from build123d import *

# Parameters (mm, degrees)
F1_DEPTH = 508
F2_W     = 80.340108
F2_H     = 50.8
F2_W_2   = 82.870346
F3_DEPTH = 12.7
F4_W     = 83.715823
F4_H     = 50.8
F4_W_2   = 80.30174
F5_DEPTH = 12.7


with BuildPart() as f1:
    # F0 (on Front) → F1 (new body)
    with BuildSketch(Plane.XZ):
        with BuildLine():
            Line((3.550242, 42.501207), (-21.849758, 42.501207))
            ThreePointArc((-21.849758, 42.501207), (-32.272509, 23.451207), (-21.849758, 4.401207))
            Line((-21.849758, 4.401207), (3.550242, 4.401207))
            ThreePointArc((3.550242, 4.401207), (13.712078, 23.451207), (3.550242, 42.501207))
        make_face()
    extrude(amount=F1_DEPTH)

    # F2 (on face) → F3 (cut)
    with BuildSketch(Plane.XY.offset(42.501207)):
        with Locations((-9.149758, -406.4)):
            Rectangle(F2_W, F2_H)
        with Locations((-9.149758, -101.6)):
            Rectangle(F2_W_2, F2_H)
    extrude(amount=-F3_DEPTH, mode=Mode.SUBTRACT)

    # F4 (on face) → F5 (cut)
    with BuildSketch(Plane(origin=(0, 0, 4.401207), x_dir=(1, 0, 0), z_dir=(0, 0, -1))):
        with Locations((-9.149757, 101.6)):
            Rectangle(F4_W, F4_H)
        with Locations((-9.149758, 406.4)):
            Rectangle(F4_W_2, F4_H)
    extrude(amount=-F5_DEPTH, mode=Mode.SUBTRACT)


solid = f1.part
CAD build for the part. Positions are in the model's coordinates, mm. A direction names the side the tool comes from. Coordinates: 2 decimals unless noted, no trailing zeros. Loops run counter-clockwise (first coordinate to the right, second up) from the corner with the lowest first, then second, coordinate; pieces in that order, holes last. Notation, with made-up numbers: (-19, 21) - (18, 21) arc R22 ccw to (18, 34) - close; hole circle Ø11 at (-5.75, -27). An arc over 180 degrees is marked (long way). Use one line per item in the form item = value. Start each with the question number.
1) Band-saw the part on B-B (y = -308). Give the cut face in (x, z).
2) Drill centre lines: L1, parallel to Y at x = 6, z = 31.5; L2, parallel to X at y = -138.5, z = 24; L3, parallel to Z at x = 10, y = -388. Where is each one in solid material? Low to high. Write a range as from..to.
3) Band-saw the part on C-C (x = -26.5). Give the cut face in (y, z), and give its area (3 significant figures).
4) Flat gauge pins, fed straight in: pin 1 (6 mm diameter, centred on y = -75, z = 15.5, fed in from -X); pin 2 (2 mm diameter, centred on y = -435, z = 37, fed in from -X); pin 3 (2 mm diameter, centred on x = -25.5, y = -107, fed in from +Z). Where does each tip first touch, or does it go through?
5) Band-saw the part on A-A (x = -1). Give the cut face in (y, z).
6) Tool access for faces 1 (the face through (-10, -406, 29.801)), 2 (the face through (-10, -127, 11)), 3 (the face through (-9, -38, 4.401)): list every direction of +Z, -Z, +X, -X, +Y, -Y with a clear straight run to the whole face (end or side of a thin tool).
Check values:
q1.outline = (-21.85, 4.4) - (3.55, 4.4) arc R22.94 ccw to (3.55, 42.5) - (-21.85, 42.5) arc R22.62 ccw to start
q2.L1 = -508..-431.8, -381..-127, -76.2..0
q2.L2 = -32.27..13.71
q2.L3 = 17.1..29.8
q3.outline = (-508, 8.36) - (-431.8, 8.36) - (-431.8, 17.1) - (-381, 17.1) - (-381, 8.36) - (-127, 8.36) - (-127, 17.1) - (-76.2, 17.1) - (-76.2, 8.36) - (0, 8.36) - (0, 38.55) - (-76.2, 38.55) - (-76.2, 29.8) - (-127, 29.8) - (-127, 38.55) - (-381, 38.55) - (-381, 29.8) - (-431.8, 29.8) - (-431.8, 38.55) - (-508, 38.55) - close
q3.area = 13,600 mm2
q4.pin_1 = -31.72
q4.pin_2 = -28.47
q4.pin_3 = 29.8
q5.outline = (-508, 4.4) - (-431.8, 4.4) - (-431.8, 17.1) - (-381, 17.1) - (-381, 4.4) - (-127, 4.4) - (-127, 17.1) - (-76.2, 17.1) - (-76.2, 4.4) - (0, 4.4) - (0, 42.5) - (-76.2, 42.5) - (-76.2, 29.8) - (-127, 29.8) - (-127, 42.5) - (-381, 42.5) - (-381, 29.8) - (-431.8, 29.8) - (-431.8, 42.5) - (-508, 42.5) - close
q6.face_1 = +Z, +X, -X
q6.face_2 = -Z, +X, -X
q6.face_3 = -Z, +X, -X, +Y, -Y
